from build123d import *

# Parameters (mm, degrees)
SKETCH_1_W      = 3.660528642
SKETCH_1_H      = 10.65279893
EXTRUDE_1_DEPTH = 3


with BuildPart() as part:
    # 草图1 → 凸台-拉伸1 (new body)
    with BuildSketch(Plane.XY.offset(3)):
        Polygon((45.580049157, 0), (45.580049157, 5.99999), (42.580009157, 5.99999), (42.580009157, 7.99949), (38.581009157, 7.99949), (38.581009157, 6.74959), (36.079809157, 6.74959), (36.079809157, 7.99949), (32.580009157, 7.99949), (32.580009157, 10.99949), (36.079809157, 10.99949), (36.079809157, 12.25079), (38.581009157, 12.25079), (38.581009157, 10.99949), (42.580009157, 10.99949), (42.580009157, 13.00039), (45.580049157, 13.00039), (45.580049157, 19.00039), (-4.419390843, 19.00039), (-4.419390843, 13.00039), (-1.419350843, 13.00039), (-1.419350843, 10.99949), (2.579649157, 10.99949), (2.579649157, 12.25079), (5.080849157, 12.25079), (5.080849157, 10.99949), (8.580649157, 10.99949), (8.580649157, 7.99949), (5.080849157, 7.99949), (5.080849157, 6.74959), (2.579649157, 6.74959), (2.579649157, 7.99949), (-1.419350843, 7.99949), (-1.419350843, 5.99999), (-4.419390843, 5.99999), (-4.419390843, 0), align=None)
        with Locations((17.524355382, 9.504123146)):
            Rectangle(SKETCH_1_W, SKETCH_1_H, mode=Mode.SUBTRACT)
    extrude(amount=-EXTRUDE_1_DEPTH)


solid = part.part
Can you work these out from the model? Positions are in its coordinate system, mm. A direction names the side the tool comes from. Coordinates: 2 decimals unless noted, no trailing zeros. Loops run counter-clockwise (first coordinate to the right, second up) from the corner with the lowest first, then second, coordinate; pieces in that order, holes last. Notation, with made-up numbers: (-39, 41.5) - (14, 41.5) arc R21 cw to (14, 53.5) - close; hole circle Ø9 at (83.25, 27). An arc over 180 degrees is marked (long way). Put each result on its own line as item: value. Start each with the question number.
Item 1: If we mould it in two halves opening along Y, with no side actions, what happens to faces 1 (the face through (19.355, 9, 2)), 2 (the face through (45.58, 3, 2))? For each: +Y half, -Y half, draft (parallel to the pull), parting line (faces both ways), or undercut.
Item 2: Suppose I cut it at A-A (y = 11.5). Please give me the cut outline in (x, z).
Item 3: If I drill on line 1 along X through (y, z) = (11.5, 2.8); line 2 along Y through (x, z) = (16, 0.2); line 3 along X through (y, z) = (14.75, 2.85), over which ranges is the centre line in solid material (lowest first)?
Item 4: Suppose I cut it at B-B (x = 4.5). Please give me the cut outline in (y, z), and give its area (3 significant figures).
Item 5: Suppose I cut it at C-C (y = 5.25). Please give me the cut outline in (x, z), and give its area (3 significant figures).
Item 6: For pin 1 (1 mm diameter, centred on y = 7.5, z = 1, fed in from -X); pin 2 (1.4 mm diameter, centred on y = 7.5, z = 1, fed in from +X), each with a flat end and sliding along its axis, tell me the tip position at first contact or that it passes through.
Item 7: Which directions (+Z, -Z, +X, -X, +Y, -Y) give clear straight access to the entire face, cutting with the end or side of a thin tool? Please do faces 3 (the face through (-4.419, 16, 2)), 4 (the face through (42.58, 7, 2)), 5 (the face through (8.581, 10, 2)), 6 (the face through (38.581, 7, 2)).
Here are the results:
1. face 1: undercut
1. face 2: draft
2. outline: (-1.42, 0) - (2.58, 0) - (2.58, 3) - (-1.42, 3) - close; (5.08, 0) - (15.69, 0) - (15.69, 3) - (5.08, 3) - close; (19.35, 0) - (36.08, 0) - (36.08, 3) - (19.35, 3) - close; (38.58, 0) - (42.58, 0) - (42.58, 3) - (38.58, 3) - close
3. line 1: -1.42 to 2.58, 5.08 to 15.69, 19.35 to 36.08, 38.58 to 42.58
3. line 2: 0 to 4.18, 14.83 to 19
3. line 3: -4.42 to 15.69, 19.35 to 45.58
4. outline: (0, 0) - (6.75, 0) - (6.75, 3) - (0, 3) - close; (12.25, 0) - (19, 0) - (19, 3) - (12.25, 3) - close
4. area: 40.5 mm²
5. outline: (-4.42, 0) - (15.69, 0) - (15.69, 3) - (-4.42, 3) - close; (19.35, 0) - (45.58, 0) - (45.58, 3) - (19.35, 3) - close
5. area: 139 mm²
6. pin 1: x = -1.42
6. pin 2: x = 42.58
7. face 3: +Z, -Z, -X, +Y, -Y
7. face 4: +Z, -Z, +X
7. face 5: +Z, -Z, -X
7. face 6: +Z, -Z
